Input: part model. Units: mm. Frame: model coordinates. Face numbers are marked on the shaded views. A direction names the side the tool comes from. Coordinates: 2 decimals unless noted, no trailing zeros. Loops run counter-clockwise (first coordinate to the right, second up) from the corner with the lowest first, then second, coordinate; pieces in that order, holes last.
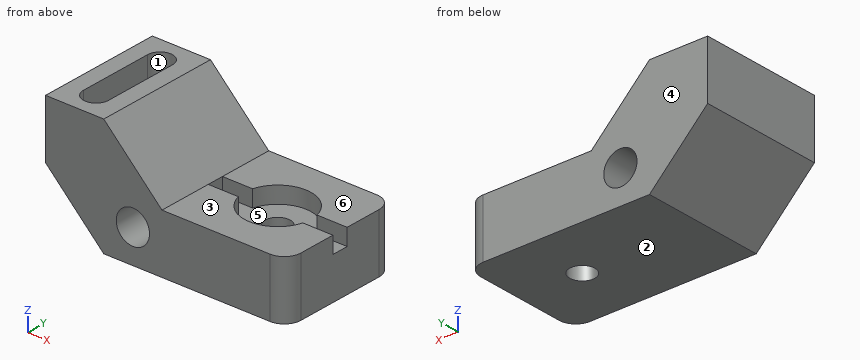
```python
from build123d import *

# Parameters (mm, degrees)
F1_DEPTH       = 38.1
F3_DEPTH       = 76.201
F4_R           = 10.16
F6_DEPTH       = 27.94
F8_D           = 15.24
F8_CBORE_D     = 40.64
F8_CBORE_DEPTH = 10.16
F10_DEPTH      = 10.16
F11_R          = 10.16
F12_DEPTH      = 76.201


with BuildPart() as f1:
    # F0 (on Front) → F1 (new body, symmetric)
    with BuildSketch(Plane.XZ):
        Polygon((0, 71.12), (0, 0), (147.32, 0), (147.32, 35.56), (71.12, 35.56), (35.56, 71.12), align=None)
    extrude(amount=F1_DEPTH, both=True)

    # F2 (on face) → F3 (cut, through all)
    with BuildSketch(Plane.XZ.offset(38.1)):
        Polygon((0, 35.56), (0, 0), (35.56, 0), align=None)
    extrude(amount=-F3_DEPTH, mode=Mode.SUBTRACT)

    # F4
    f4_edges = [f1.edges().sort_by_distance(p)[0] for p in [
        (147.32, -38.1, 17.78),
        (147.32, 38.1, 17.78),
    ]]
    fillet(f4_edges, radius=F4_R)

    # F5 (on face) → F6 (cut)
    with BuildSketch(Plane.XY.offset(71.12)):
        with BuildLine():
            ThreePointArc((25.4, 22.86), (17.78, 30.48), (10.16, 22.86))
            Line((10.16, 22.86), (10.16, -22.86))
            ThreePointArc((10.16, -22.86), (17.78, -30.48), (25.4, -22.86))
            Line((25.4, -22.86), (25.4, 22.86))
        make_face()
    extrude(amount=-F6_DEPTH, mode=Mode.SUBTRACT)

    # F8 (through all)
    with Locations(Plane.XY.offset(35.56)):
        with Locations((109.22, 0)):
            CounterBoreHole(F8_D / 2, F8_CBORE_D / 2, F8_CBORE_DEPTH)

    # F9 (on face) → F10 (cut)
    with BuildSketch(Plane.XY.offset(35.56)):
        Polygon((71.12, 5.08), (71.12, 0), (71.12, -5.08), (147.32, -5.08), (147.32, 0), (147.32, 5.08), align=None)
    extrude(amount=-F10_DEPTH, mode=Mode.SUBTRACT)

    # F11 (on face) → F12 (cut, through all)
    with BuildSketch(Plane.XZ.offset(38.1)):
        with Locations((53.34, 20.32)):
            Circle(F11_R)
    extrude(amount=-F12_DEPTH, mode=Mode.SUBTRACT)


solid = f1.part
```
Item 1: Section query C-C (x = 109.22). Output: boundary loops of the cut face in (y, z).
Result:
outline: (-38.1, 0) - (-7.62, 0) - (-7.62, 25.4) - (-20.32, 25.4) - (-20.32, 35.56) - (-38.1, 35.56) - close; (7.62, 0) - (38.1, 0) - (38.1, 35.56) - (20.32, 35.56) - (20.32, 25.4) - (7.62, 25.4) - close
Item 2: Section query D-D (z = 33). Output: boundary loops of the cut face in (x, y), then the cut area to 3 significant figures.
Result:
outline: (2.56, -38.1) - (137.16, -38.1) arc R10.16 ccw to (147.32, -27.94) - (147.32, -5.08) - (128.89, -5.08) arc R20.32 cw to (89.55, -5.08) - (71.12, -5.08) - (71.12, 5.08) - (89.55, 5.08) arc R20.32 cw to (128.89, 5.08) - (147.32, 5.08) - (147.32, 27.94) arc R10.16 ccw to (137.16, 38.1) - (2.56, 38.1) - close
area: 9,320 mm2
Item 3: Contact query for flat-ended pins moving along their axis: P1, Ø6, axis at y = -23.5, z = 61.5, coming from the +X side; P2, Ø10, axis at x = 43.5, y = 14, coming from the +Z side; P3, Ø10, axis at x = 20, y = -2, coming from the +Z side; P4, Ø18.5, axis at x = 53.34, z = 20.32, coming from the -Y side. Output: stop coordinate, or through.
Result:
P1: stops at x = 48.18
P2: stops at z = 68.18
P3: stops at z = 43.18
P4: passes through
Item 4: Section query B-B (z = 20.32). Output: boundary loops of the cut face in (x, y), then the cut area to 3 significant figures.
Result:
outline: (15.24, -38.1) - (43.18, -38.1) - (43.18, 38.1) - (15.24, 38.1) - close; (63.5, -38.1) - (137.16, -38.1) arc R10.16 ccw to (147.32, -27.94) - (147.32, 27.94) arc R10.16 ccw to (137.16, 38.1) - (63.5, 38.1) - close; hole circle Ø15.24 at (109.22, 0)
area: 8,290 mm2
Item 5: Reachability of the marked faces 1, 2 and 3 from +Z, -Z, +X, -X, +Y, -Y: full face, straight path, thin tool, end or side. Return the list, or none.
Result:
face 1: +Z
face 2: -Z, +X, -X, +Y, -Y
face 3: +Z, +X, +Y, -Y
Item 6: Mould query, pull axis Y, two halves, no side actions, for the marked faces 4, 5 and 6. Classes: +Y half, -Y half, draft (parallel to the pull), parting line (faces both ways), or undercut.
Result:
face 4: +Y half
face 5: undercut
face 6: draft
Item 7: Section query A-A (y = 0). Output: boundary loops of the cut face in (x, z), then the cut area to 3 significant figures.
Result:
outline: (0, 35.56) - (35.56, 0) - (101.6, 0) - (101.6, 25.4) - (71.12, 25.4) - (71.12, 35.56) - (35.56, 71.12) - (25.4, 71.12) - (25.4, 43.18) - (10.16, 43.18) - (10.16, 71.12) - (0, 71.12) - close; (116.84, 0) - (147.32, 0) - (147.32, 25.4) - (116.84, 25.4) - close; hole circle Ø20.32 at (53.34, 20.32)
area: 4,590 mm2
Item 8: Line query: L1, parallel to Y at x = 136.5, z = 27; L2, parallel to Y at x = 109.22, z = 19.5; L3, parallel to X at y = -0.5, z = 23. Output: solid intervals per line, ascending.
Result:
L1: y = -38.1 to -5.08, 5.08 to 38.1
L2: y = -38.1 to -7.62, 7.62 to 38.1
L3: x = 12.56 to 43.54, 63.14 to 101.62, 116.82 to 147.32
